Geometry: see drawing. Coordinates: mm, zero at the bounding-box minimum. A direction names the side the tool comes from. Give positions to 0.01 mm unless a question says otherwise; leave off trailing zeros. Write each loop counter-clockwise with the first axis right and the second up, starting at its lowest first coordinate (ties: lowest second). Pieces come first, ordered by that corner, then holes. Notation, with made-up numbers: (77.5, 16) -> (121.5, 16) arc R27 ccw to (121.5, 35) -> close; hole circle Ø2 at (84.25, -36.75). An arc over 180 degrees is marked (long way). Use one line per item in the form item = value. Start each with the question number.
(1) Draft query along X for the marked faces 4, 5 and 6. Return one class per face: pulls with the +X half, pulls with the -X half, needs draft (parallel to the pull), parting line crosses it, or undercut.
(2) Set-up query: the marked faces 1, 2 and 3. Return all of +Z, -Z, +X, -X, +Y, -Y with unobstructed straight access to the full face (end or side cutting, diameter ignored); none if empty.
(3) Cut plane C-C, the plane z = 13. Output: boundary loops of the cut face in (x, y).
(4) Cut plane A-A, the plane y = 21. Output: boundary loops of the cut face in (x, z), and give its area (3 significant figures).
(5) Cut plane D-D, the plane x = 33. Output: boundary loops of the cut face in (y, z), and give its area (3 significant figures).
(6) Material intervals for line 1 along X through (y, z) = (6, 6) (1 decimal); line 2 along Y through (x, z) = (36, 2.25); line 3 along X through (y, z) = (3, 2.25) (1 decimal), sorted ascending. Write a range as from..to.
(7) First-contact query: P1, Ø9, axis at x = 36.5, y = 8, coming from the -Z side; P2, Ø4, axis at x = 7, y = 7.5, coming from the -Z side; P3, Ø1, axis at y = 11.5, z = 11.5, coming from the -X side; P4, Ø7, axis at x = 35.85, y = 6.15, coming from the +Z side. Flat tips, straight axial feed; report the tip coordinate or a pass-through.
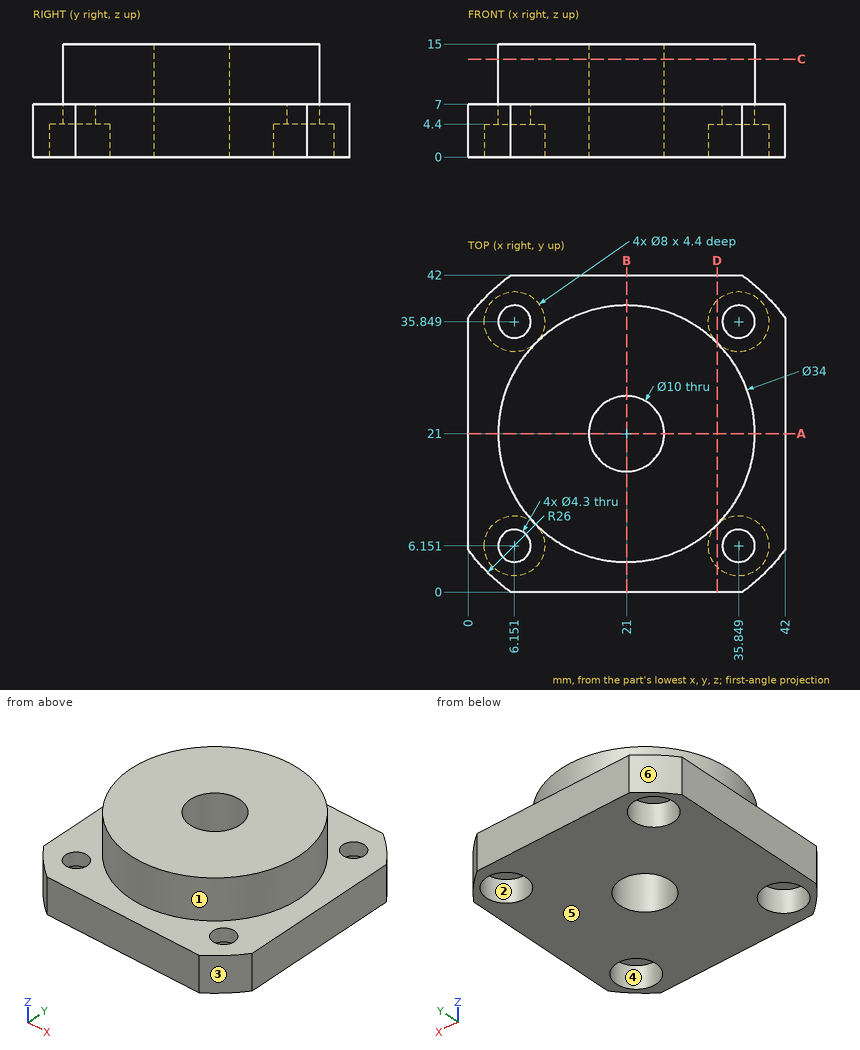
Geometry says:
q1.face_4 = undercut
q1.face_5 = needs draft
q1.face_6 = pulls with the -X half
q2.face_1 = +Z
q2.face_2 = -Z
q2.face_3 = +Z, -Z, +X, -Y
q3.outline = circle Ø34 at (21, 21); hole circle Ø10 at (21, 21)
q4.outline = (0, 0) -> (16, 0) -> (16, 15) -> (4, 15) -> (4, 7) -> (0, 7) -> close; (26, 0) -> (42, 0) -> (42, 7) -> (38, 7) -> (38, 15) -> (26, 15) -> close
q4.area = 416 mm^2
q5.outline = (0, 0) -> (3.34, 0) -> (3.34, 4.4) -> (8.96, 4.4) -> (8.96, 0) -> (33.04, 0) -> (33.04, 4.4) -> (38.66, 4.4) -> (38.66, 0) -> (42, 0) -> (42, 7) -> (33.04, 7) -> (33.04, 15) -> (8.96, 15) -> (8.96, 7) -> (0, 7) -> close
q5.area = 437 mm^2
q6.line_1 = 0..4, 8.3..33.7, 38..42
q6.line_2 = 0..2.15, 10.15..31.85, 39.85..42
q6.line_3 = 2.2..3.7, 8.6..33.4, 38.3..39.8
q7.P1 = 0
q7.P2 = 4.4
q7.P3 = 6.58
q7.P4 = 7
